Input: part model. Units: mm. Frame: model coordinates. Face numbers are marked on the shaded views. A direction names the side the tool comes from. Coordinates: 2 decimals unless noted, no trailing zeros. Write each loop counter-clockwise with the first axis right and the second up, starting at its lowest first coordinate (ties: lowest second). Pieces come first, ordered by that corner, then holes.
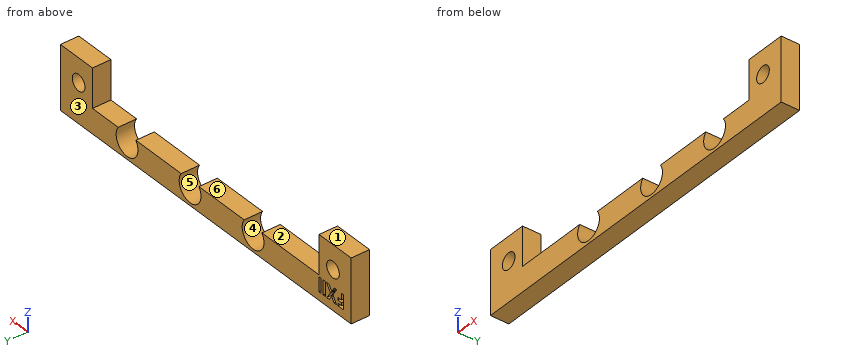
from build123d import *

# Parameters (mm, degrees)
BOSS_EXTRUDE1_OUTLINE_R = 1.75
BOSS_EXTRUDE1_DEPTH     = 4
SKETCH2_W               = 0.569871794
SKETCH2_H               = 3.175
SKETCH2_W_2             = 0.569871795
CUT_EXTRUDE1_DEPTH      = 1


# Read off the part's stored shape, not the designer's step: Boss-Extrude1
with BuildPart() as part:
    # Boss-Extrude1 outline → Boss-Extrude1 (new body)
    with BuildSketch(Plane(origin=(0, 0, 0), x_dir=(1, 0, 0), z_dir=(0, 1, 0))):
        with BuildLine():
            Line((25.076474615, -10.33744254), (37.54307775, -10.33744254))
            ThreePointArc((37.54307775, -10.33744254), (39.979776182, -5.587442326), (42.416474615, -10.33744254))
            Line((42.416474615, -10.33744254), (49.479776182, -10.33744254))
            Line((49.479776182, -10.33744254), (49.479776182, -18.81631662))
            Line((49.479776182, -18.81631662), (58.304776182, -18.81631662))
            Line((58.304776182, -18.81631662), (58.304776182, -4.977921711))
            Line((58.304776182, -4.977921711), (-21.695223818, -4.977921711))
            Line((-21.695223818, -4.977921711), (-21.695223818, -18.81631662))
            Line((-21.695223818, -18.81631662), (-12.870223818, -18.81631662))
            Line((-12.870223818, -18.81631662), (-12.870223818, -10.33744254))
            Line((-12.870223818, -10.33744254), (2.86307775, -10.33744254))
            ThreePointArc((2.86307775, -10.33744254), (5.299776182, -5.587442326), (7.736474615, -10.33744254))
            Line((7.736474615, -10.33744254), (20.20307775, -10.33744254))
            ThreePointArc((20.20307775, -10.33744254), (22.639776183, -5.587442326), (25.076474615, -10.33744254))
        make_face()
        with Locations((-16.695223818, -13.587442433)):
            Circle(BOSS_EXTRUDE1_OUTLINE_R, mode=Mode.SUBTRACT)
        with Locations((53.304776182, -13.587442433)):
            Circle(BOSS_EXTRUDE1_OUTLINE_R, mode=Mode.SUBTRACT)
    extrude(amount=BOSS_EXTRUDE1_DEPTH)

    # Sketch2 → Cut-Extrude1 (cut)
    with BuildSketch(Plane(origin=(0, 4, 0), x_dir=(1, 0, 0), z_dir=(0, 1, 0))):
        Polygon((-19.588408787, -6.762736227), (-18.041613915, -6.762736227), (-18.041613915, -7.332608022), (-19.018536992, -7.332608022), (-19.018536992, -7.943184945), (-18.041613915, -7.943184945), (-18.041613915, -8.51305674), (-19.018536992, -8.51305674), (-19.018536992, -9.937736227), (-19.588408787, -9.937736227), align=None)
        Polygon((-17.665727497, -6.762736227), (-16.994092881, -6.762736227), (-16.330726495, -7.782272485), (-15.666088073, -6.762736227), (-14.992545405, -6.762736227), (-15.99427317, -8.298718799), (-14.927671607, -9.937736227), (-15.599306223, -9.937736227), (-16.330726495, -8.813893078), (-17.063418803, -9.937736227), (-17.736325453, -9.937736227), (-16.666543803, -8.297446764), align=None)
        with Locations((-14.29674212, -8.350236227)):
            Rectangle(SKETCH2_W, SKETCH2_H)
        with Locations((-13.075588274, -8.350236227)):
            Rectangle(SKETCH2_W_2, SKETCH2_H)
    extrude(amount=-CUT_EXTRUDE1_DEPTH, mode=Mode.SUBTRACT)


solid = part.part
Item 1: Section query C-C, the plane x = 31. Return loops of the section in (y, z), then the cut area to 3 significant figures.
Item 2: Section query A-A, the plane z = 17. Return loops of the section in (x, y), then the cut area to 3 significant figures.
Item 3: Material intervals for line 1 (X direction, y = 1.8, z = 8.5); line 2 (X direction, y = 3, z = 11); line 3 (X direction, y = 0.8, z = 13.25), sorted ascending.
Item 4: Pull-direction query (Z, two-part tool) for the marked faces 3, 4, 5 and 6; classes: released by +Z, released by -Z, zero draft, split by the parting line, or undercut.
Item 5: Access query for the marked faces 1 and 2. Directions: +Z, -Z, +X, -X, +Y, -Y. A direction counts if a zero-diameter tool reaches every point of the face in a straight line with its end or side. Return the directions, or none.
Item 6: Section query B-B, the plane y = 1.7. Return loops of the section in (x, z), then the cut area to 3 significant figures.
Item 7: Pin query (flat end, axial travel): pin 1 Ø2 at (x, y) = (31, 1.5) entering from +Z. Return the tip coordinate at first contact, or that it passes through.
The answers:
1. outline: (0, 4.98) - (4, 4.98) - (4, 10.34) - (0, 10.34) - close
1. area: 21.4 mm2
2. outline: (-21.7, 0) - (-12.87, 0) - (-12.87, 4) - (-21.7, 4) - close; (49.48, 0) - (58.3, 0) - (58.3, 4) - (49.48, 4) - close
2. area: 70.6 mm2
3. line 1: x = -21.7 to 2.3, 8.3 to 19.64, 25.64 to 36.98, 42.98 to 58.3
3. line 2: x = -21.7 to -12.87, 49.48 to 58.3
3. line 3: x = -21.7 to -18.41, -14.98 to -12.87, 49.48 to 51.59, 55.02 to 58.3
4. face 3: zero draft
4. face 4: undercut
4. face 5: undercut
4. face 6: released by +Z
5. face 1: +Z, +X, -X, +Y, -Y
5. face 2: +Z, +Y, -Y
6. outline: (-21.7, 4.98) - (58.3, 4.98) - (58.3, 18.82) - (49.48, 18.82) - (49.48, 10.34) - (42.42, 10.34) arc R3 cw (long way) to (37.54, 10.34) - (25.08, 10.34) arc R3 cw (long way) to (20.2, 10.34) - (7.74, 10.34) arc R3 cw (long way) to (2.86, 10.34) - (-12.87, 10.34) - (-12.87, 18.82) - (-21.7, 18.82) - close; hole circle Ø3.5 at (-16.7, 13.59); hole circle Ø3.5 at (53.3, 13.59)
6. area: 487 mm2
7. pin 1: stops at z = 10.34
